```python
from build123d import *

# Parameters (mm, degrees)
SKETCH2_W               = 115
SKETCH2_H               = 110
BOSS_EXTRUDE1_DEPTH     = 2
CUT_EXTRUDE1_DEPTH      = 80.594283714
CUT_EXTRUDE1_DEPTH_BACK = 80.594283714
SKETCH3_W               = 90
SKETCH3_H               = 57
SKETCH4_W               = 10
SKETCH4_H               = 10
CUT_EXTRUDE2_DEPTH      = 2
SKETCH5_W               = 78
SKETCH5_H               = 8
CUT_EXTRUDE3_DEPTH      = 80.594283714
SKETCH6_W               = 78.002684591
SKETCH6_H               = 3.125
BOSS_EXTRUDE3_DEPTH     = 10
BOSS_EXTRUDE6_DEPTH     = 10
SKETCH10_W              = 2
SKETCH10_H              = 8
BOSS_EXTRUDE7_DEPTH     = 12
SKETCH11_W              = 2
SKETCH11_H              = 8
BOSS_EXTRUDE8_DEPTH     = 12
SKETCH12_W              = 15
SKETCH12_H              = 3
BOSS_EXTRUDE9_DEPTH     = 10
SKETCH13_W              = 15
SKETCH13_H              = 3
BOSS_EXTRUDE10_DEPTH    = 10
SKETCH14_W              = 74
SKETCH14_H              = 8
BOSS_EXTRUDE11_DEPTH    = 2
SKETCH17_R              = 2.375
CUT_EXTRUDE4_DEPTH      = 81.195074662
SKETCH18_W              = 10
SKETCH18_H              = 10
BOSS_EXTRUDE12_DEPTH    = 2
CUT_EXTRUDE5_DEPTH      = 81.468938107
CUT_EXTRUDE5_DEPTH_BACK = 81.468938107
SKETCH20_W              = 10
SKETCH20_H              = 10


with BuildPart() as part:
    # Sketch2 → Boss-Extrude1 (new body)
    with BuildSketch(Plane(origin=(0, 0, 0), x_dir=(1, 0, 0), z_dir=(0, 1, 0))):
        Rectangle(SKETCH2_W, SKETCH2_H)
    extrude(amount=BOSS_EXTRUDE1_DEPTH)

    # Sketch3 → Cut-Extrude1 (cut, two sides: drawn at the far end of the back side and taken through both)
    with BuildSketch(Plane(origin=(0, 2, 0), x_dir=(1, 0, 0), z_dir=(0, 1, 0)).offset(-CUT_EXTRUDE1_DEPTH_BACK)):
        with Locations((-5, -12)):
            Rectangle(SKETCH3_W, SKETCH3_H)
    extrude(amount=CUT_EXTRUDE1_DEPTH + CUT_EXTRUDE1_DEPTH_BACK, mode=Mode.SUBTRACT)

    # Sketch4 → Cut-Extrude2 (cut)
    with BuildSketch(Plane(origin=(0, 2, 0), x_dir=(1, 0, 0), z_dir=(0, 1, 0))):
        with Locations((-5, 35.75)):
            Rectangle(SKETCH4_W, SKETCH4_H)
    extrude(amount=-CUT_EXTRUDE2_DEPTH, mode=Mode.SUBTRACT)

    # Sketch5 → Cut-Extrude3 (cut, through all)
    with BuildSketch(Plane(origin=(0, 2, 0), x_dir=(1, 0, 0), z_dir=(0, 1, 0))):
        with Locations((-5, 23.625)):
            Rectangle(SKETCH5_W, SKETCH5_H)
    extrude(amount=-CUT_EXTRUDE3_DEPTH, mode=Mode.SUBTRACT)

    # Sketch6 → Boss-Extrude3 (add)
    with BuildSketch(Plane(origin=(0, 0, 0), x_dir=(-1, 0, 0), z_dir=(0, -1, 0))):
        with Locations((4.998657704, 18.0625)):
            Rectangle(SKETCH6_W, SKETCH6_H)
    extrude(amount=BOSS_EXTRUDE3_DEPTH)

    # Sketch8 → Boss-Extrude6 (add)
    with BuildSketch(Plane(origin=(0, 0, 0), x_dir=(-1, 0, 0), z_dir=(0, -1, 0))):
        Polygon((-34, 28.625), (-34, 27.625), (-32, 27.625), (42, 27.625), (44, 27.625), (44, 28.625), (29, 28.625), (-19, 28.625), align=None)
    extrude(amount=BOSS_EXTRUDE6_DEPTH)

    # Sketch10 → Boss-Extrude7 (add)
    with BuildSketch(Plane(origin=(0, 2, 0), x_dir=(1, 0, 0), z_dir=(0, 1, 0))):
        with Locations((33, 23.625)):
            Rectangle(SKETCH10_W, SKETCH10_H)
    extrude(amount=-BOSS_EXTRUDE7_DEPTH)

    # Sketch11 → Boss-Extrude8 (add)
    with BuildSketch(Plane(origin=(0, 2, 0), x_dir=(1, 0, 0), z_dir=(0, 1, 0))):
        with Locations((-43, 23.625)):
            Rectangle(SKETCH11_W, SKETCH11_H)
    extrude(amount=-BOSS_EXTRUDE8_DEPTH)

    # Sketch12 → Boss-Extrude9 (add)
    with BuildSketch(Plane(origin=(0, 0, 0), x_dir=(-1, 0, 0), z_dir=(0, -1, 0))):
        with Locations((-26.5, 30.125)):
            Rectangle(SKETCH12_W, SKETCH12_H)
    extrude(amount=BOSS_EXTRUDE9_DEPTH)

    # Sketch13 → Boss-Extrude10 (add)
    with BuildSketch(Plane(origin=(0, 0, 0), x_dir=(-1, 0, 0), z_dir=(0, -1, 0))):
        with Locations((36.5, 30.125)):
            Rectangle(SKETCH13_W, SKETCH13_H)
    extrude(amount=BOSS_EXTRUDE10_DEPTH)

    # Sketch14 → Boss-Extrude11 (add)
    with BuildSketch(Plane(origin=(0, -10, 0), x_dir=(-1, 0, 0), z_dir=(0, -1, 0))):
        with Locations((5, 23.625)):
            Rectangle(SKETCH14_W, SKETCH14_H)
    extrude(amount=-BOSS_EXTRUDE11_DEPTH)

    # Sketch17 → Cut-Extrude4 (cut, through all)
    with BuildSketch(Plane(origin=(0, -8, 0), x_dir=(1, 0, 0), z_dir=(0, 1, 0))):
        with Locations(Location((25, 23.625, 0), (0, 0, 270))):
            Circle(SKETCH17_R)
        with Locations(Location((-35, 23.625, 0), (0, 0, 270))):
            Circle(SKETCH17_R)
        with Locations(Location((-26.43, 23.625, 0), (0, 0, 270))):
            Circle(SKETCH17_R)
        with Locations(Location((-17.86, 23.625, 0), (0, 0, 270))):
            Circle(SKETCH17_R)
        with Locations(Location((-0.72, 23.625, 0), (0, 0, 270))):
            Circle(SKETCH17_R)
        with Locations(Location((7.85, 23.625, 0), (0, 0, 270))):
            Circle(SKETCH17_R)
        with Locations(Location((16.42, 23.625, 0), (0, 0, 270))):
            Circle(SKETCH17_R)
        with Locations(Location((-9.29, 23.625, 0), (0, 0, 270))):
            Circle(SKETCH17_R)
    extrude(amount=-CUT_EXTRUDE4_DEPTH, mode=Mode.SUBTRACT)

    # Sketch18 → Boss-Extrude12 (add)
    with BuildSketch(Plane(origin=(0, 2, 0), x_dir=(1, 0, 0), z_dir=(0, 1, 0))):
        with Locations((-5, 35.75)):
            Rectangle(SKETCH18_W, SKETCH18_H)
    extrude(amount=-BOSS_EXTRUDE12_DEPTH)

    # Sketch20 → Cut-Extrude5 (cut, two sides: drawn at the far end of the back side and taken through both)
    with BuildSketch(Plane(origin=(0, 2, 0), x_dir=(1, 0, 0), z_dir=(0, 1, 0)).offset(-CUT_EXTRUDE5_DEPTH_BACK)):
        with Locations((-5, 41.5)):
            Rectangle(SKETCH20_W, SKETCH20_H)
    extrude(amount=CUT_EXTRUDE5_DEPTH + CUT_EXTRUDE5_DEPTH_BACK, mode=Mode.SUBTRACT)


solid = part.part
```
Read the model definition and answer for the solid it produces. Units are mm, in the model's axes. A direction names the side the tool comes from. Give positions to 0.01 mm unless a question says otherwise; leave off trailing zeros. Write each loop counter-clockwise with the first axis right and the second up, starting at its lowest first coordinate (ties: lowest second). Pieces come first, ordered by that corner, then holes. Notation, with made-up numbers: (34.25, 11) -> (59.25, 11) arc R11 ccw to (59.25, 22) -> close; hole circle Ø8 at (-10, 42). An arc over 180 degrees is marked (long way). Answer as a JSON object with one key per item and string values.
1) Flat-ended cylindrical pins translate along their axes: pin 1 Ø4 at (x, z) = (-26.43, -23.625) entering from +Y; pin 2 Ø3.5 at (x, y) = (2, -6) entering from +Z; pin 3 Ø2 at (x, y) = (-43.5, -8) entering from -Z (3 decimals); pin 4 Ø2.5 at (y, z) = (-7.5, -18) entering from +X. Find the tip coordinate at first contact, or state that the pin passes through.
Findings below:
{"pin 1": "passes through", "pin 2": "stops at z = -16.5", "pin 3": "stops at z = -31.625", "pin 4": "stops at x = 34"}
2) A tool of negligible diameter and unlimited length cuts with its end or side. For faces 5 (the flat face through (34.003, -5, -18)), 6 (the flat face through (32, -3, -24)), 7 (the flat face through (27, -5, -31.625)), from which of +Z, -Z, +X, -X, +Y, -Y can it reach the whole face along a straight path? Write none if from no direction.
Findings below:
{"face 5": "+Z, -Z, +X, -Y", "face 6": "+Y", "face 7": "-Z, +X, -X, -Y"}
3) Section D-D on x = -47.5 is taken. Write down the section's boundary in (y, z).
Findings below:
{"outline": "(0, -55) -> (2, -55) -> (2, -16.5) -> (0, -16.5) -> close; (0, 40.5) -> (2, 40.5) -> (2, 55) -> (0, 55) -> close"}
4) Section C-C on z = -5.5 is taken. Write down the section's boundary in (x, y), then the cut area to 3 significant figures.
Findings below:
{"outline": "(-57.5, 0) -> (-50, 0) -> (-50, 2) -> (-57.5, 2) -> close; (40, 0) -> (57.5, 0) -> (57.5, 2) -> (40, 2) -> close", "area": "50.0 mm^2"}
5) Straight lines are drawn through the part: probe 1 along Z at (x, y) = (0.5, 1) (3 decimals); probe 2 along Z at (x, y) = (12.5, -2) (3 decimals); probe 3 along Y at (x, z) = (37, -31). For each, find the intervals that lie inside material, in ascending order. Write a range as from..to.
Findings below:
{"probe 1": "z = -55..-27.625, -19.625..-16.5, 40.5..55", "probe 2": "z = -28.625..-27.625, -19.625..-16.5", "probe 3": "y = 0..2"}
6) For a pull along X with two mould halves and no side action, classify faces 1 (the flat face through (34, -5, -26)), 2 (the flat face through (12, 2, -37)), 3 (the cylindrical face through (-10.735, -8.986, -25.51)), 4 (the flat face through (-44, -5, -24)) as pulls with the +X half, pulls with the -X half, needs draft (parallel to the pull), parting line crosses it, or undercut.
Findings below:
{"face 1": "pulls with the +X half", "face 2": "needs draft", "face 3": "undercut", "face 4": "pulls with the -X half"}
7) Section A-A on x = -22.5 is taken. Write down the section's boundary in (y, z) (3 decimals), then the cut area to 3 significant figures.
Findings below:
{"outline": "(-10, -28.625) -> (0, -28.625) -> (0, -55) -> (2, -55) -> (2, -27.625) -> (-8, -27.625) -> (-8, -19.625) -> (2, -19.625) -> (2, -16.5) -> (-10, -16.5) -> close; (0, 40.5) -> (2, 40.5) -> (2, 55) -> (0, 55) -> close", "area": "147 mm^2"}
